from build123d import *

# Parameters (mm, degrees)
SKETCH1_R           = 2.7
BOSS_EXTRUDE1_DEPTH = 5
SKETCH2_R           = 7.5
BOSS_EXTRUDE2_DEPTH = 15
BOSS_EXTRUDE3_DEPTH = 3.5


with BuildPart() as part:
    # Sketch1 → Boss-Extrude1 (new body)
    # profile 1 of 4: a face of its own
    with BuildSketch(Plane.XY):
        with BuildLine():
            Line((0, 89.8), (0, 85))
            ThreePointArc((0, 85), (60.104076401, 60.104076401), (85, 0))
            Line((85, 0), (89.8, 0))
            ThreePointArc((89.8, 0), (92.5, 2.7), (95.2, 0))
            Line((95.2, 0), (100, 0))
            ThreePointArc((100, 0), (70.710678119, 70.710678119), (0, 100))
            Line((0, 100), (0, 95.2))
            ThreePointArc((0, 95.2), (1.909188309, 94.409188309), (2.7, 92.5))
            ThreePointArc((2.7, 92.5), (1.909188309, 90.590811691), (0, 89.8))
        make_face()
        with Locations((90.722638437, 18.045854786)):
            Circle(SKETCH1_R, mode=Mode.SUBTRACT)
        with Locations((85.458856757, 35.398217494)):
            Circle(SKETCH1_R, mode=Mode.SUBTRACT)
        with Locations((18.045854786, 90.722638437)):
            Circle(SKETCH1_R, mode=Mode.SUBTRACT)
        with Locations((35.398217494, 85.458856757)):
            Circle(SKETCH1_R, mode=Mode.SUBTRACT)
        with Locations((65.40737726, 65.40737726)):
            Circle(SKETCH1_R, mode=Mode.SUBTRACT)
        with Locations((76.910939138, 51.390246554)):
            Circle(SKETCH1_R, mode=Mode.SUBTRACT)
        with Locations((51.390246554, 76.910939138)):
            Circle(SKETCH1_R, mode=Mode.SUBTRACT)
    # profile 2 of 4: a face of its own
    with BuildSketch(Plane.XY):
        with BuildLine():
            ThreePointArc((85, 0), (60.104076401, -60.104076401), (0, -85))
            Line((0, -85), (0, -89.8))
            ThreePointArc((0, -89.8), (1.909188309, -90.590811691), (2.7, -92.5))
            ThreePointArc((2.7, -92.5), (1.909188309, -94.409188309), (0, -95.2))
            Line((0, -95.2), (0, -100))
            ThreePointArc((0, -100), (70.710678119, -70.710678119), (100, 0))
            Line((100, 0), (95.2, 0))
            ThreePointArc((95.2, 0), (92.5, -2.7), (89.8, 0))
            Line((89.8, 0), (85, 0))
        make_face()
        with Locations((18.045854786, -90.722638437)):
            Circle(SKETCH1_R, mode=Mode.SUBTRACT)
        with Locations((35.398217494, -85.458856757)):
            Circle(SKETCH1_R, mode=Mode.SUBTRACT)
        with Locations((51.390246554, -76.910939138)):
            Circle(SKETCH1_R, mode=Mode.SUBTRACT)
        with Locations((65.40737726, -65.40737726)):
            Circle(SKETCH1_R, mode=Mode.SUBTRACT)
        with Locations((76.910939138, -51.390246554)):
            Circle(SKETCH1_R, mode=Mode.SUBTRACT)
        with Locations((85.458856757, -35.398217494)):
            Circle(SKETCH1_R, mode=Mode.SUBTRACT)
        with Locations((90.722638437, -18.045854786)):
            Circle(SKETCH1_R, mode=Mode.SUBTRACT)
    # profile 3 of 4: a face of its own
    with BuildSketch(Plane.XY):
        with BuildLine():
            ThreePointArc((0, -85), (-60.104076401, -60.104076401), (-85, 0))
            Line((-85, 0), (-89.8, 0))
            ThreePointArc((-89.8, 0), (-92.5, -2.7), (-95.2, 0))
            Line((-95.2, 0), (-100, 0))
            ThreePointArc((-100, 0), (-70.710678119, -70.710678119), (0, -100))
            Line((0, -100), (0, -95.2))
            ThreePointArc((0, -95.2), (-2.7, -92.5), (0, -89.8))
            Line((0, -89.8), (0, -85))
        make_face()
        with Locations((-51.390246554, -76.910939138)):
            Circle(SKETCH1_R, mode=Mode.SUBTRACT)
        with Locations((-76.910939138, -51.390246554)):
            Circle(SKETCH1_R, mode=Mode.SUBTRACT)
        with Locations((-65.40737726, -65.40737726)):
            Circle(SKETCH1_R, mode=Mode.SUBTRACT)
        with Locations((-35.398217494, -85.458856757)):
            Circle(SKETCH1_R, mode=Mode.SUBTRACT)
        with Locations((-18.045854786, -90.722638437)):
            Circle(SKETCH1_R, mode=Mode.SUBTRACT)
        with Locations((-85.458856757, -35.398217494)):
            Circle(SKETCH1_R, mode=Mode.SUBTRACT)
        with Locations((-90.722638437, -18.045854786)):
            Circle(SKETCH1_R, mode=Mode.SUBTRACT)
    # profile 4 of 4: a face of its own
    with BuildSketch(Plane.XY):
        with BuildLine():
            Line((-89.8, 0), (-85, 0))
            ThreePointArc((-85, 0), (-60.104076401, 60.104076401), (0, 85))
            Line((0, 85), (0, 89.8))
            ThreePointArc((0, 89.8), (-2.7, 92.5), (0, 95.2))
            Line((0, 95.2), (0, 100))
            ThreePointArc((0, 100), (-70.710678119, 70.710678119), (-100, 0))
            Line((-100, 0), (-95.2, 0))
            ThreePointArc((-95.2, 0), (-92.5, 2.7), (-89.8, 0))
        make_face()
        with Locations((-90.722638437, 18.045854786)):
            Circle(SKETCH1_R, mode=Mode.SUBTRACT)
        with Locations((-85.458856757, 35.398217494)):
            Circle(SKETCH1_R, mode=Mode.SUBTRACT)
        with Locations((-76.910939138, 51.390246554)):
            Circle(SKETCH1_R, mode=Mode.SUBTRACT)
        with Locations((-65.40737726, 65.40737726)):
            Circle(SKETCH1_R, mode=Mode.SUBTRACT)
        with Locations((-51.390246554, 76.910939138)):
            Circle(SKETCH1_R, mode=Mode.SUBTRACT)
        with Locations((-35.398217494, 85.458856757)):
            Circle(SKETCH1_R, mode=Mode.SUBTRACT)
        with Locations((-18.045854786, 90.722638437)):
            Circle(SKETCH1_R, mode=Mode.SUBTRACT)
    extrude(amount=BOSS_EXTRUDE1_DEPTH)



with BuildPart() as body_2:
    # Sketch2 → Boss-Extrude2 (new body)
    with BuildSketch(Plane.XY):
        Circle(SKETCH2_R)
        with BuildLine():
            Line((-1.997498436, 2.5), (1.997498436, 2.5))
            ThreePointArc((1.997498436, 2.5), (0, -3.2), (-1.997498436, 2.5))
        make_face(mode=Mode.SUBTRACT)
    extrude(amount=BOSS_EXTRUDE2_DEPTH)


with BuildPart() as part_1:
    add(part.part)

    add(body_2.part)  # Boss-Extrude3 merges body 2
    # Sketch3 → Boss-Extrude3 (add)
    with BuildSketch(Plane.XY):
        with BuildLine():
            Line((84.976467331, 2), (7.228416147, 2))
            ThreePointArc((7.228416147, 2), (7.5, 0), (7.228416147, -2))
            Line((7.228416147, -2), (84.976467331, -2))
            ThreePointArc((84.976467331, -2), (85, 0), (84.976467331, 2))
        make_face()
        with BuildLine():
            Line((44.220284473, -72.591779432), (5.346258881, -5.259992013))
            ThreePointArc((5.346258881, -5.259992013), (3.75, -6.495190528), (1.882157266, -7.259992013))
            Line((1.882157266, -7.259992013), (40.756182858, -74.591779432))
            ThreePointArc((40.756182858, -74.591779432), (42.5, -73.612159322), (44.220284473, -72.591779432))
        make_face()
        with BuildLine():
            Line((-40.756182858, -74.591779432), (-1.882157266, -7.259992013))
            ThreePointArc((-1.882157266, -7.259992013), (-3.75, -6.495190528), (-5.346258881, -5.259992013))
            Line((-5.346258881, -5.259992013), (-44.220284473, -72.591779432))
            ThreePointArc((-44.220284473, -72.591779432), (-42.5, -73.612159322), (-40.756182858, -74.591779432))
        make_face()
        with BuildLine():
            Line((-84.976467331, -2), (-7.228416147, -2))
            ThreePointArc((-7.228416147, -2), (-7.5, 0), (-7.228416147, 2))
            Line((-7.228416147, 2), (-84.976467331, 2))
            ThreePointArc((-84.976467331, 2), (-85, 0), (-84.976467331, -2))
        make_face()
        with BuildLine():
            Line((-44.220284473, 72.591779432), (-5.346258881, 5.259992013))
            ThreePointArc((-5.346258881, 5.259992013), (-3.75, 6.495190528), (-1.882157266, 7.259992013))
            Line((-1.882157266, 7.259992013), (-40.756182858, 74.591779432))
            ThreePointArc((-40.756182858, 74.591779432), (-42.5, 73.612159322), (-44.220284473, 72.591779432))
        make_face()
        with BuildLine():
            Line((40.756182858, 74.591779432), (1.882157266, 7.259992013))
            ThreePointArc((1.882157266, 7.259992013), (3.75, 6.495190528), (5.346258881, 5.259992013))
            Line((5.346258881, 5.259992013), (44.220284473, 72.591779432))
            ThreePointArc((44.220284473, 72.591779432), (42.5, 73.612159322), (40.756182858, 74.591779432))
        make_face()
    extrude(amount=BOSS_EXTRUDE3_DEPTH)


solid = part_1.part
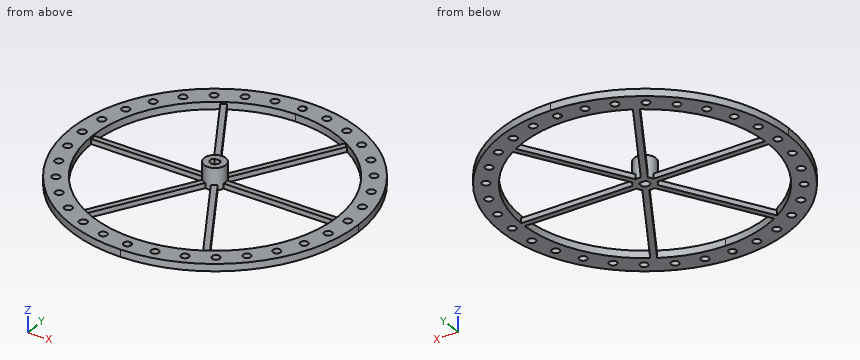
Geometry: final body of the model. Coordinates: model frame, mm. Give positions to 0.01 mm unless a question says otherwise; leave off trailing zeros. Write each loop counter-clockwise with the first axis right and the second up, starting at its lowest first coordinate (ties: lowest second). Pieces come first, ordered by that corner, then holes. Notation, with made-up numbers: (23.5, 7) -> (36.5, 7) arc R24 ccw to (36.5, 29) -> close; hole circle Ø8 at (87, 32.5). An arc over 180 degrees is marked (long way). Answer as a JSON object with one key per item and string values.
1. Contact query for flat-ended pins moving along their axis: pin 1 (5 mm diameter, centred on x = -51.39, y = -76.91, fed in from -Z); pin 2 (8.5 mm diameter, centred on x = 65.41, y = 65.41, fed in from +Z); pin 3 (1 mm diameter, centred on x = 54.5, z = 4, fed in from -Y); pin 4 (5 mm diameter, centred on x = -35, z = 5, fed in from -Y). Output: stop coordinate, or through.
Ans:
{"pin 1": "passes through", "pin 2": "stops at z = 5", "pin 3": "stops at y = -84.17", "pin 4": "stops at y = -94.57"}
2. Ray query, probe 1 along X at (y, z) = (34.5, 3.25); probe 2 along X at (y, z) = (85.5, 1.75); probe 3 along Y at (x, z) = (92.5, 3). Return the intervals inside material, ascending. Write a range as from..to.
Ans:
{"probe 1": "x = -93.86..-88.01, -82.91..-77.68, -22.23..-17.61, 17.61..22.23, 77.68..82.91, 88.01..93.86", "probe 2": "x = -51.86..-38.1, -32.7..32.7, 38.1..51.86", "probe 3": "y = -38..-20.08, -16.01..-2.7, 2.7..16.01, 20.08..38"}
3. Cut plane A-A on y = 23.5. Output: boundary loops of the cut face in (x, z).
Ans:
{"outline": "(-97.2, 0) -> (-81.69, 0) -> (-81.69, 5) -> (-97.2, 5) -> close; (-15.88, 0) -> (-11.26, 0) -> (-11.26, 3.5) -> (-15.88, 3.5) -> close; (11.26, 0) -> (15.88, 0) -> (15.88, 3.5) -> (11.26, 3.5) -> close; (81.69, 0) -> (97.2, 0) -> (97.2, 5) -> (81.69, 5) -> close"}
4. Cut plane B-B on z = 7.25. Output: boundary loops of the cut face in (x, y), and give its area (3 significant figures).
Ans:
{"outline": "circle Ø15 at (0, 0); hole (-2, 2.5) arc R3.2 ccw (long way) to (2, 2.5) -> close", "area": "146 mm^2"}
